Here's the drawing with two shaded views (mm, measured from the low corner). I have some questions. Coordinates: 2 decimals unless noted, no trailing zeros. Order: outer loops, then holes, each group sorted by start corner. A loop starts at its lowest first (then second) coordinate and runs counter-clockwise, first axis right, second up. Notation, with made-up numbers: (69, 84.25) -> (80, 84.25) arc R23 ccw to (80, 93.25) -> close; hole circle Ø1 at (24, 82). An arc over 180 degrees is marked (long way). Answer as a JSON object with one key per item and string values. Group by question number.
(1) I want a section at B-B, the plane y = 1. List the corners of the cut face in (x, z) for me.
(2) I need wall thicknesses on line 1 (X direction, y = 5, z = 6.15); line 2 (X direction, y = 1.1, z = 6.15). Which ranges of each line are inside material? Lowest first, please.
(3) I want a section at D-D, the plane x = 21.15. List the corners of the cut face in (y, z) for me.
(4) If we mould it in two halves opening along X, with no side actions, what happens to the marked faces 1, 2 and 3? For each: pulls with the +X half, pulls with the -X half, needs draft (parallel to the pull), parting line crosses it, or undercut.
(5) I want a section at A-A, the plane z = 36.15. List the corners of the cut face in (x, y) for me.
(6) I want a section at C-C, the plane x = 36.15. List the corners of the cut face in (y, z) for me, plus the area to 3 significant figures.
(7) For pin 1 (3 mm diameter, centred on x = 36.5, z = 6, fed in from -Y); pin 2 (1 mm diameter, centred on x = 30.5, z = 20.5, fed in from +Y), each with a flat end and sliding along its axis, tell me the tip position at first contact or that it passes through.
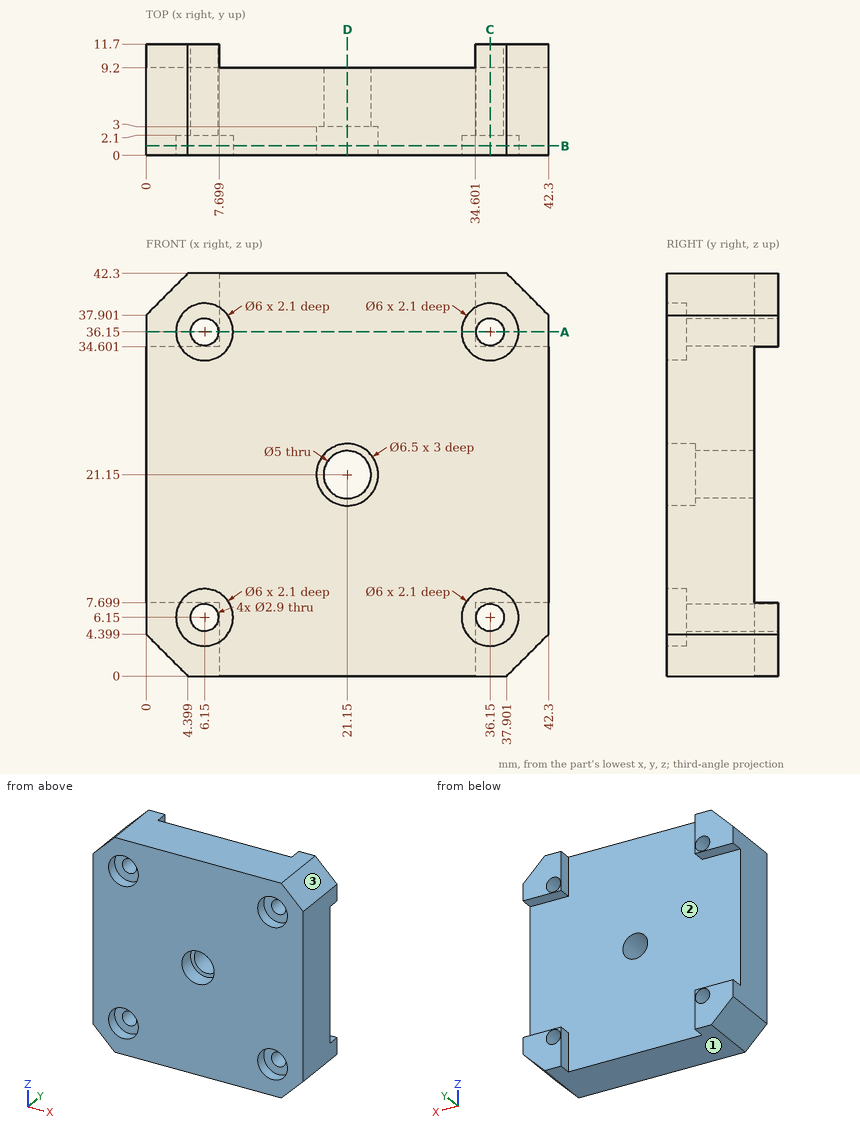
Computed values:
{
 "1": {"outline": "(0, 4.4) -> (4.4, 0) -> (37.9, 0) -> (42.3, 4.4) -> (42.3, 37.9) -> (37.9, 42.3) -> (4.4, 42.3) -> (0, 37.9) -> close; hole circle Ø6 at (6.15, 6.15); hole circle Ø6 at (6.15, 36.15); hole circle Ø6.5 at (21.15, 21.15); hole circle Ø6 at (36.15, 6.15); hole circle Ø6 at (36.15, 36.15)"},
 "2": {"line 1": "x = 0 to 4.7, 7.6 to 34.7, 37.6 to 42.3", "line 2": "x = 0 to 3.15, 9.15 to 33.15, 39.15 to 42.3"},
 "3": {"outline": "(0, 0) -> (9.2, 0) -> (9.2, 18.65) -> (3, 18.65) -> (3, 17.9) -> (0, 17.9) -> close; (0, 24.4) -> (3, 24.4) -> (3, 23.65) -> (9.2, 23.65) -> (9.2, 42.3) -> (0, 42.3) -> close"},
 "4": {"face 1": "needs draft", "face 2": "undercut", "face 3": "pulls with the +X half"},
 "5": {"outline": "(0, 0) -> (3.15, 0) -> (3.15, 2.1) -> (4.7, 2.1) -> (4.7, 11.7) -> (0, 11.7) -> close; (7.6, 2.1) -> (9.15, 2.1) -> (9.15, 0) -> (33.15, 0) -> (33.15, 2.1) -> (34.7, 2.1) -> (34.7, 11.7) -> (34.6, 11.7) -> (34.6, 9.2) -> (7.7, 9.2) -> (7.7, 11.7) -> (7.6, 11.7) -> close; (37.6, 2.1) -> (39.15, 2.1) -> (39.15, 0) -> (42.3, 0) -> (42.3, 11.7) -> (37.6, 11.7) -> close"},
 "6": {"outline": "(0, 0) -> (11.7, 0) -> (11.7, 4.7) -> (2.1, 4.7) -> (2.1, 3.15) -> (0, 3.15) -> close; (0, 9.15) -> (2.1, 9.15) -> (2.1, 7.6) -> (11.7, 7.6) -> (11.7, 7.7) -> (9.2, 7.7) -> (9.2, 34.6) -> (11.7, 34.6) -> (11.7, 34.7) -> (2.1, 34.7) -> (2.1, 33.15) -> (0, 33.15) -> close; (0, 39.15) -> (2.1, 39.15) -> (2.1, 37.6) -> (11.7, 37.6) -> (11.7, 42.3) -> (0, 42.3) -> close", "area": "347 mm2"},
 "7": {"pin 1": "stops at y = 2.1", "pin 2": "stops at y = 9.2"}
}
